For this review, take the finished solid that the model builds, in its own axes (mm). A direction names the side the tool comes from. Round coordinates to 2 decimals unless told otherwise and drop trailing zeros. Loops run counter-clockwise (first coordinate to the right, second up) from the corner with the lowest first, then second, coordinate; pieces in that order, holes last.
```python
from build123d import *

# Parameters (mm, degrees)
SKETCH1_R            = 80
BOSS_EXTRUDE1_DEPTH  = 15
SKETCH16_R           = 10
BOSS_EXTRUDE2_DEPTH  = 200
FILLET1_R            = 10
CUT_SWEEP2_PROFILE_R = 4.7625


with BuildPart() as part:
    # Sketch1 → Boss-Extrude1 (new body)
    with BuildSketch(Plane(origin=(0, 0, 0), x_dir=(1, 0, 0), z_dir=(0, 1, 0))):
        Circle(SKETCH1_R)
    extrude(amount=BOSS_EXTRUDE1_DEPTH)

    # Sketch16 → Boss-Extrude2 (add)
    with BuildSketch(Plane(origin=(0, 15, 0), x_dir=(1, 0, 0), z_dir=(0, 1, 0))):
        Circle(SKETCH16_R)
    extrude(amount=BOSS_EXTRUDE2_DEPTH)

    # Fillet1
    fillet1_edges = [part.edges().sort_by_distance(p)[0] for p in [
        (-10, 15, 0),
    ]]
    fillet(fillet1_edges, radius=FILLET1_R)

    # Cut-Sweep2: sweep along a path in Sketch29
    with BuildLine(Plane(origin=(0, 18, 0), x_dir=(1, 0, 0), z_dir=(0, 1, 0))) as cut_sweep2_path:
        CenterArc((0, 0), 50, 0, 360)
    # Cut-Sweep2 profile (on start of the path) → Cut-Sweep2 (sweep, cut)
    with BuildSketch(Plane(origin=(50, 18, 0), x_dir=(-1, 0, 0), z_dir=(0, 0, -1))):
        Circle(CUT_SWEEP2_PROFILE_R)
    sweep(path=cut_sweep2_path.line, mode=Mode.SUBTRACT)


solid = part.part
```
(1) Add section C-C (y = 109.5). Give the boundary of the cut face in (x, z).
(2) Add section B-B (x = 0). Give the boundary of the cut face in (y, z) (1 decimal), plus the area to 3 significant figures.
(3) Add section D-D (y = 17.5). Give the boundary of the cut face in (x, z).
(4) Insertion check: pin 1 Ø10 at (x, y) = (-11.5, 104) entering from -Z; pin 2 Ø3 at (x, z) = (36, 31.5) entering from +Y; pin 3 Ø1 at (x, z) = (-56.5, 57.5) entering from +Y. Each pin has a flat end and moves straight along its axis. Give the tip position at first contact, or say it passes through.
(5) Add section A-A (z = 0). Give the boundary of the cut face in (x, y) (1 decimal), plus the area to 3 significant figures.
(6) For faces 1 (the flat face through (-1, 0, -1)), 2 (the flat face through (10, 15, 20)), list the 3-axis set-ups (+Z, -Z, +X, -X, +Y, -Y) from which the entire face can be reached by the end or side of a thin tool; tool diameter is ignored.
(7) For L1, parallel to Y at x = 48, z = -35.5; L2, parallel to Y at x = -41, z = 22; L3, parallel to X at y = 9, z = 16, list the stretches that pass through material, from the lowest coordinate up.
Outcome:
1. outline: circle Ø20 at (0, 0)
2. outline: (0, -80) - (15, -80) - (15, -53.7) arc R4.8 cw to (15, -46.3) - (15, -20) arc R10 cw to (25, -10) - (215, -10) - (215, 10) - (25, 10) arc R10 cw to (15, 20) - (15, 46.3) arc R4.8 cw to (15, 53.7) - (15, 80) - (0, 80) - close
2. area: 6,420 mm2
3. outline: circle Ø26.77 at (0, 0)
4. pin 1: stops at z = -7.6
4. pin 2: stops at y = 14.96
4. pin 3: passes through
5. outline: (-80, 0) - (80, 0) - (80, 15) - (53.7, 15) arc R4.8 cw to (46.3, 15) - (20, 15) arc R10 cw to (10, 25) - (10, 215) - (-10, 215) - (-10, 25) arc R10 cw to (-20, 15) - (-46.3, 15) arc R4.8 cw to (-53.7, 15) - (-80, 15) - close
5. area: 6,420 mm2
6. face 1: +Z, -Z, +X, -X, -Y
6. face 2: +Y
7. L1: y = 0 to 15
7. L2: y = 0 to 14.74
7. L3: x = -78.38 to 78.38
